Can you work these out from the drawing? Everything is in mm from the part's minimum corner. Give positions to 0.01 mm unless a question says otherwise; leave off trailing zeros. Order: outer loops, then holes, each group sorted by start corner. A loop starts at its lowest first (then second) coordinate and runs counter-clockwise, first axis right, second up. Notation, with made-up numbers: M 28.25,59 L 58.25,59 A21 cw 58.25,66 Z; hole C 82,23 d2. An arc over 180 degrees is marked long. Use a Markdown table: item, result. Add a question column.
Item 1: I'm going to push flat-ended pins straight in: pin 1 Ø0.5 at (y, z) = (1, 9) entering from -X; pin 2 Ø0.7 at (x, z) = (1.5, 9.5) entering from +Y. Where does each tip first touch, or does it pass through?
Item 2: If I drill on L1, parallel to Z at x = 1, y = 0.25; L2, parallel to Y at x = 1, z = 4; L3, parallel to X at y = 0.1, z = 7, over which ranges is the centre line in solid material (lowest first)? Write a range as from..to.
Item 3: Suppose I cut it at A-A on z = 7.25. Write out the boundary of the cut face in (x, y), plus the area to 3 significant figures.
Item 4: Suppose I cut it at C-C on x = 0.45. Write out the boundary of the cut face in (y, z), plus the area to 3 significant figures.
Item 5: Suppose I cut it at B-B on y = 1.3. Write out the boundary of the cut face in (x, z), plus the area to 4 significant figures.
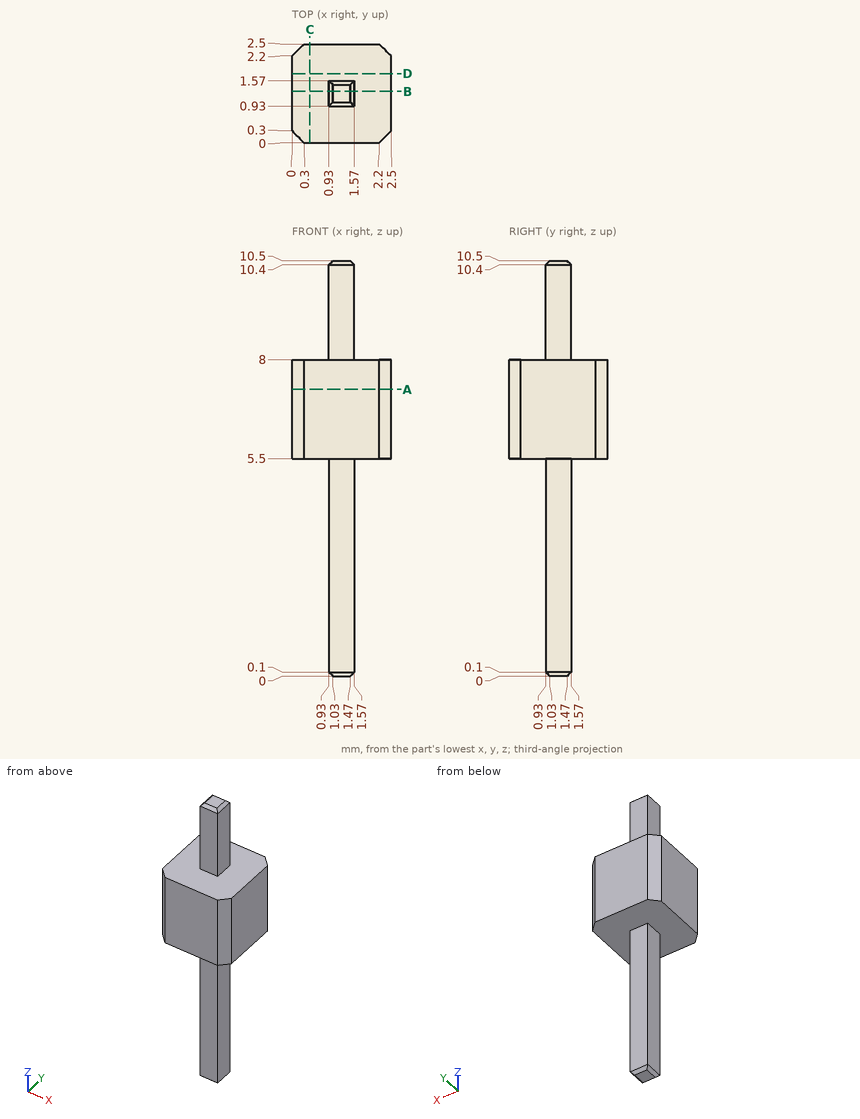
Findings below:
| question | item | result |
|---|---|---|
| 1 | pin 1 | stops at x = 0.93 |
| 1 | pin 2 | stops at y = 1.57 |
| 2 | L1 | z = 5.5..8 |
| 2 | L2 | y = 0.93..1.57 |
| 2 | L3 | x = 0.2..2.3 |
| 3 | outline | M 0,0.3 L 0.3,0 L 2.2,0 L 2.5,0.3 L 2.5,2.2 L 2.2,2.5 L 0.3,2.5 L 0,2.2 Z |
| 3 | area | 6.07 mm^2 |
| 4 | outline | M 0,5.5 L 2.5,5.5 L 2.5,8 L 0,8 Z |
| 4 | area | 6.25 mm^2 |
| 5 | outline | M 0,5.5 L 0.93,5.5 L 0.93,0.1 L 1.03,0 L 1.47,0 L 1.57,0.1 L 1.57,5.5 L 2.5,5.5 L 2.5,8 L 1.57,8 L 1.57,10.4 L 1.47,10.5 L 1.03,10.5 L 0.93,10.4 L 0.93,8 L 0,8 Z |
| 5 | area | 11.35 mm^2 |
